from build123d import *

# Parameters (mm, degrees)
F0_W     = 298.45
F0_H     = 203.2
F0_R     = 4.031729
F1_DEPTH = 4.445
F0_H_2   = 12.7
F2_DEPTH = 3.175


with BuildPart() as f1:
    # F0 (on Front) → F1 (new body)
    with BuildSketch(Plane.XZ):
        Rectangle(F0_W, F0_H)
        with Locations((-137.795, -76.2)):
            Circle(F0_R, mode=Mode.SUBTRACT)
        with Locations((137.795, -76.2)):
            Circle(F0_R, mode=Mode.SUBTRACT)
        with Locations((-137.795, 76.2)):
            Circle(F0_R, mode=Mode.SUBTRACT)
        with Locations((137.795, 76.2)):
            Circle(F0_R, mode=Mode.SUBTRACT)
    extrude(amount=F1_DEPTH)

    # F0 (on Front) → F2 (join)
    with BuildSketch(Plane.XZ):
        with Locations((0, 107.95)):
            Rectangle(F0_W, F0_H_2)
        Rectangle(F0_W, F0_H)
        with Locations((-137.795, -76.2)):
            Circle(F0_R, mode=Mode.SUBTRACT)
        with Locations((137.795, -76.2)):
            Circle(F0_R, mode=Mode.SUBTRACT)
        with Locations((-137.795, 76.2)):
            Circle(F0_R, mode=Mode.SUBTRACT)
        with Locations((137.795, 76.2)):
            Circle(F0_R, mode=Mode.SUBTRACT)
        with Locations((0, -107.95)):
            Rectangle(F0_W, F0_H_2)
    extrude(amount=-F2_DEPTH)


solid = f1.part
Input: part model. Units: mm. Frame: model coordinates. A direction names the side the tool comes from. Coordinates: 2 decimals unless noted, no trailing zeros. Order: outer loops, then holes, each group sorted by start corner. A loop starts at its lowest first (then second) coordinate and runs counter-clockwise, first axis right, second up. Notation, with made-up numbers: M 22,-25.5 L 53,-25.5 A19 ccw 53,-19.5 Z; hole C -35.5,57.25 d11. An arc over 180 degrees is marked long. Write item = value, one per line. Start each with the question number.
(1) Reachability of faces 1 (the flat face through (-2, 0, -108)), 2 (the flat face through (-2, -4.445, 1)), 3 (the flat face through (-2, 0, 108)) from +Z, -Z, +X, -X, +Y, -Y: full face, straight path, thin tool, end or side. Return the list, or none.
(2) Line query: line 1 along X through (y, z) = (-1.25, 77) (3 decimals); line 2 along Z through (x, y) = (-119.5, -2.75). Output: solid intervals per line, ascending. Write a range as [from, to].
(3) Section A-A on z = 76.2. Output: boundary loops of the cut face in (x, y) (3 decimals), and give its area (3 significant figures).
(4) Section C-C on x = -125. Output: boundary loops of the cut face in (y, z) (3 decimals), and give its area (3 significant figures).
(5) Section B-B on y = -1.5. Output: boundary loops of the cut face in (x, z) (3 decimals), and give its area (3 significant figures).
(6) First-contact query: P1, Ø6.5, axis at x = -137.795, z = 76.2, coming from the +Y side; P2, Ø2, axis at x = -57.5, y = -3.5, coming from the +Z side; P3, Ø6.5, axis at x = 24.5, z = -109.5, coming from the -Y side. Flat tips, straight axial feed; report the tip coordinate or a pass-through.
Result set:
q1.face_1 = -Z, +X, -X, -Y
q1.face_2 = +Z, -Z, +X, -X, -Y
q1.face_3 = +Z, +X, -X, -Y
q2.line_1 = [-149.225, -141.747], [-133.843, 133.843], [141.747, 149.225]
q2.line_2 = [-101.6, 101.6]
q3.outline = M -149.225,-4.445 L -141.827,-4.445 L -141.827,3.175 L -149.225,3.175 Z; M -133.763,-4.445 L 133.763,-4.445 L 133.763,3.175 L -133.763,3.175 Z; M 141.827,-4.445 L 149.225,-4.445 L 149.225,3.175 L 141.827,3.175 Z
q3.area = 2,150 mm²
q4.outline = M -4.445,-101.6 L 0,-101.6 L 0,-114.3 L 3.175,-114.3 L 3.175,114.3 L 0,114.3 L 0,101.6 L -4.445,101.6 Z
q4.area = 1,630 mm²
q5.outline = M -149.225,-101.6 L 149.225,-101.6 L 149.225,101.6 L -149.225,101.6 Z; hole C -137.795,-76.2 d8.063; hole C -137.795,76.2 d8.063; hole C 137.795,-76.2 d8.063; hole C 137.795,76.2 d8.063
q5.area = 60,400 mm²
q6.P1 = through
q6.P2 = 101.6
q6.P3 = 0
